```python
from build123d import *

# Parameters (mm, degrees)
ESQUISSE4_OUTSIDE_W     = 35.66
ESQUISSE4_OUTSIDE_H     = 35.66
ESQUISSE4_OUTSIDE_W_2   = 31.580909768
ESQUISSE4_OUTSIDE_H_2   = 22
ENL_V_MAT_EXTRU_1_DEPTH = 10
ESQUISSE5_R             = 5.937171044
BOSS_EXTRU_1_DEPTH      = 10
ESQUISSE6_R             = 3
BOSS_EXTRU_2_DEPTH      = 11


with BuildPart() as part:
    # Esquisse1 → Révolution1 (revolve)
    with BuildSketch(Plane.XY):
        with BuildLine():
            Line((0, -23.183892617), (0, 1.816107383))
            ThreePointArc((0, 1.816107383), (-12.5, -10.683892617), (0, -23.183892617))
        make_face()
    revolve(axis=Axis((0, -23.183892617, 0), (0, 1, 0)))

    # Esquisse4 outside → Enlèv. mat.-Extru.1 (cut)
    with BuildSketch(Plane.XY):
        with Locations((0, -10.684)):
            Rectangle(ESQUISSE4_OUTSIDE_W, ESQUISSE4_OUTSIDE_H)
        with Locations((-0.692114094, -10.683892617)):
            Rectangle(ESQUISSE4_OUTSIDE_W_2, ESQUISSE4_OUTSIDE_H_2, mode=Mode.SUBTRACT)
    enl_v_mat_extru_1 = extrude(amount=-ENL_V_MAT_EXTRU_1_DEPTH, mode=Mode.SUBTRACT)

    # Symétrie1: Enlèv. mat.-Extru.1 across plane
    add(enl_v_mat_extru_1.mirror(Plane.XY), mode=Mode.SUBTRACT)

    # Esquisse5 → Boss.-Extru.1 (add)
    with BuildSketch(Plane(origin=(0, 0.316107383, 0), x_dir=(1, 0, 0), z_dir=(0, 1, 0))):
        with Locations(Location((0, 0, 0), (0, 0, 180))):
            Circle(ESQUISSE5_R)
    extrude(amount=BOSS_EXTRU_1_DEPTH)

    # Esquisse6 → Boss.-Extru.2 (add)
    with BuildSketch(Plane(origin=(0, 10.316107383, 0), x_dir=(1, 0, 0), z_dir=(0, 1, 0))):
        with Locations(Location((0, 0, 0), (0, 0, 180))):
            Circle(ESQUISSE6_R)
    extrude(amount=BOSS_EXTRU_2_DEPTH)


solid = part.part
```
Part model, mm, in its own coordinate system. A direction names the side the tool comes from. Coordinates: 2 decimals unless noted, no trailing zeros. Write each loop counter-clockwise with the first axis right and the second up, starting at its lowest first coordinate (ties: lowest second). Pieces come first, ordered by that corner, then holes.
Item 1: Probe line 1 (X direction, y = 2, z = -2); line 2 (Y direction, x = 10, z = -5.25); line 3 (X direction, y = -17, z = -7). List the from-to ranges inside material, lowest first.
Item 2: Slice it at C-C (y = 13.5). Write the cut outline in (x, z).
Item 3: Slice it at A-A (z = 0). Write the cut outline in (x, y), and give its area (3 significant figures).
Item 4: Slice it at B-B (x = 0). Write the cut outline in (y, z), and give its area (3 significant figures).
Item 5: Pin check, flat tips, straight feed: pin 1 (1.5 mm diameter, centred on y = 0.5, z = -2.5, fed in from -X); pin 2 (10 mm diameter, centred on x = 3.5, y = -3, fed in from -Z); pin 3 (4 mm diameter, centred on x = -10, z = 1.5, fed in from -Y). Stop position of each tip, or through.
Item 6: Which spindle directions (+Z, -Z, +X, -X, +Y, -Y) get a long thin tool onto all of the face, cutting with end or side? Do faces 1 (the face through (-2.86, 15.74, 0.9)), 2 (the face through (0, 21.316, 0)). Say none if no direction does.
Item 7: Slice it at D-D (y = 7). Write the cut outline in (x, z).
Results found:
1. line 1: x = -5.59 to 5.59
1. line 2: y = -16.04 to -5.33
1. line 3: x = -8.21 to 8.21
2. outline: circle Ø6 at (0, 0)
3. outline: (-5.94, -21.68) - (5.94, -21.68) arc R12.5 ccw to (5.94, 0.32) - (5.94, 10.32) - (3, 10.32) - (3, 21.32) - (-3, 21.32) - (-3, 10.32) - (-5.94, 10.32) - (-5.94, 0.32) arc R12.5 ccw to start
3. area: 652 mm2
4. outline: (-21.68, -5.94) arc R12.5 ccw to (0.32, -5.94) - (10.32, -5.94) - (10.32, -3) - (21.32, -3) - (21.32, 3) - (10.32, 3) - (10.32, 5.94) - (0.32, 5.94) arc R12.5 ccw to (-21.68, 5.94) - close
4. area: 652 mm2
5. pin 1: stops at x = -6.45
5. pin 2: stops at z = -12.02
5. pin 3: stops at y = -20.19
6. face 1: +Y
6. face 2: +Z, -Z, +X, -X, +Y
7. outline: circle Ø11.87 at (0, 0)
